```python
from build123d import *

# Parameters (mm, degrees)
SKIZZE1_W                       = 58
SKIZZE1_H                       = 31
AUFSATZ_LINEAR_AUSTRAGEN1_DEPTH = 12
VERRUNDUNG1_R                   = 2
VERRUNDUNG2_R                   = 3
SKIZZE3_R                       = 0.875
SKIZZE3_R_2                     = 0.8
AUFSATZ_LINEAR_AUSTRAGEN2_DEPTH = 2


with BuildPart() as part:
    # Skizze1 → Aufsatz-Linear austragen1 (new body)
    with BuildSketch(Plane.XY):
        with Locations((29, 15.5)):
            Rectangle(SKIZZE1_W, SKIZZE1_H)
    extrude(amount=AUFSATZ_LINEAR_AUSTRAGEN1_DEPTH)

    # Verrundung1
    verrundung1_edges = [part.edges().sort_by_distance(p)[0] for p in [
        (58, 15.5, 12),
        (58, 15.5, 0),
    ]]
    fillet(verrundung1_edges, radius=VERRUNDUNG1_R)

    # Verrundung2
    verrundung2_edges = [part.edges().sort_by_distance(p)[0] for p in [
        (0, 15.5, 12),
        (0, 15.5, 0),
    ]]
    fillet(verrundung2_edges, radius=VERRUNDUNG2_R)

    # Skizze3 → Aufsatz-Linear austragen2 (add)
    with BuildSketch(Plane(origin=(58, 0, 0), x_dir=(0, 0, -1), z_dir=(1, 0, 0))):
        with Locations(Location((-9, 30, 0), (0, 0, 180))):
            Circle(SKIZZE3_R)
        with Locations(Location((-3, 30, 0), (0, 0, 180))):
            Circle(SKIZZE3_R)
        with Locations(Location((-4, 28.2, 0), (0, 0, 180))):
            Circle(SKIZZE3_R_2)
        with Locations(Location((-5.65, 28.2, 0), (0, 0, 180))):
            Circle(SKIZZE3_R_2)
        with Locations(Location((-7.3, 28.2, 0), (0, 0, 180))):
            Circle(SKIZZE3_R_2)
    extrude(amount=AUFSATZ_LINEAR_AUSTRAGEN2_DEPTH)


solid = part.part
```
Could you check a few things on this model? Use its own coordinates, in mm. A direction names the side the tool comes from. Give positions to 0.01 mm unless a question says otherwise; leave off trailing zeros. Loops run counter-clockwise (first coordinate to the right, second up) from the corner with the lowest first, then second, coordinate; pieces in that order, holes last. Notation, with made-up numbers: (-22, -38) - (35, -38) arc R19 cw to (35, -23) - close; hole circle Ø4 at (45.25, 34.25). An arc over 180 degrees is marked (long way). Use one line per item in the form item = value.
1. I'm going to push a flat-ended pin straight in: pin 1 Ø6 at (y, z) = (8, 8.5) entering from +X. Where does the tip first touch, or does it pass through?
Response values:
pin_1 = 58
2. On a 3-axis mill with a long thin cutter (end or side, diameter ignored), from which of +Z, -Z, +X, -X, +Y, -Y can I reach the whole of each face in a straight line? I mean faces 1 (the face through (59, 29, 4)), 2 (the face through (60, 30, 9)). Say none if no direction works.
Response values:
face_1 = +X
face_2 = +Z, -Z, +X, +Y, -Y
3. I want a section at A-A (y = 30). Please give me the cut outline in (x, z) (3 decimals).
Response values:
outline = (0, 3) arc R3 ccw to (3, 0) - (56, 0) arc R2 ccw to (58, 2) - (58, 2.125) - (60, 2.125) - (60, 3.875) - (58, 3.875) - (58, 8.125) - (60, 8.125) - (60, 9.875) - (58, 9.875) - (58, 10) arc R2 ccw to (56, 12) - (3, 12) arc R3 ccw to (0, 9) - close
4. I want a section at C-C (y = 24.5). Please give me the cut outline in (x, z), and give its area (3 significant figures).
Response values:
outline = (0, 3) arc R3 ccw to (3, 0) - (56, 0) arc R2 ccw to (58, 2) - (58, 10) arc R2 ccw to (56, 12) - (3, 12) arc R3 ccw to (0, 9) - close
area = 690 mm²
5. I want a section at B-B (z = 5.65). Please give me the cut outline in (x, y), and give its area (3 significant figures).
Response values:
outline = (0, 0) - (58, 0) - (58, 27.4) - (60, 27.4) - (60, 29) - (58, 29) - (58, 31) - (0, 31) - close
area = 1,800 mm²
6. I need wall thicknesses on probe 1 along X at (y, z) = (14.5, 4.5); probe 2 along X at (y, z) = (25.5, 10). Which ranges of each line are inside material? Lowest first, please.
Response values:
probe_1 = 0 to 58
probe_2 = 0.17 to 58
7. Thinking about a two-plate mould opening in Z: for faces 3 (the face through (60, 28, 6)), 4 (the face through (0.9, 15.72, 11.14)), 5 (the face through (58.99, 28.98, 5.48)), which applies, released by +Z, released by -Z, zero draft, split by the parting line, or undercut?
Response values:
face_3 = zero draft
face_4 = released by +Z
face_5 = undercut
